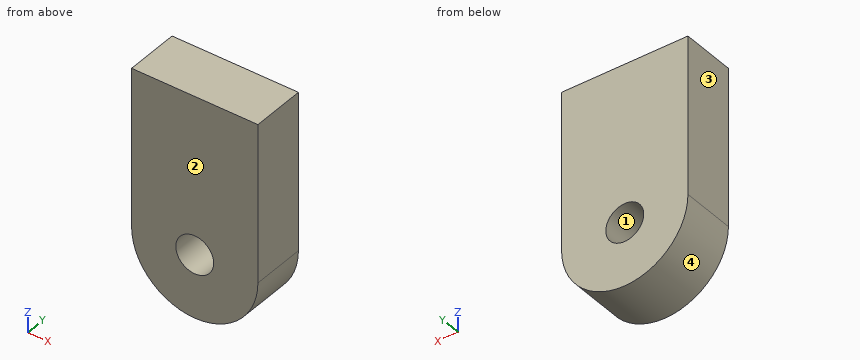
```python
from build123d import *

# Parameters (mm, degrees)
SKETCH1_R           = 2.1
BOSS_EXTRUDE1_DEPTH = 6


with BuildPart() as part:
    # Sketch1 → Boss-Extrude1 (new body)
    with BuildSketch(Plane(origin=(0, 0, 0), x_dir=(1, 0, 0), z_dir=(0, 1, 0))):
        with BuildLine():
            Line((-7, -8.75), (7, -8.75))
            Line((7, -8.75), (7, 8.75))
            ThreePointArc((7, 8.75), (0, 15.75), (-7, 8.75))
            Line((-7, 8.75), (-7, -8.75))
        make_face()
        with Locations((0, 8.75)):
            Circle(SKETCH1_R, mode=Mode.SUBTRACT)
    extrude(amount=BOSS_EXTRUDE1_DEPTH)


solid = part.part
```
For this review, take the finished solid that the model builds, in its own axes (mm). Face numbers are marked on the shaded views. Round coordinates to 2 decimals unless told otherwise and drop trailing zeros. Write each loop counter-clockwise with the first axis right and the second up, starting at its lowest first coordinate (ties: lowest second). Pieces come first, ordered by that corner, then holes. Notation, with made-up numbers: (-11, -14.5) -> (-5, -14.5) arc R31 ccw to (-5, 11.5) -> close; hole circle Ø2 at (-17, -40). An arc over 180 degrees is marked (long way). One line per question, with ' | ' between items. Start each with the question number.
1) Add section D-D (x = -4). Write out the cut boundary in (y, z).
2) Add section A-A (x = 0). Write out the cut boundary in (y, z).
3) Mouldability with a two-part tool opening along X and no side actions: class the marked faces 1, 2, 3 and 4 as +X half, -X half, draft (parallel to the pull), parting line (faces both ways), or undercut.
4) Add section C-C (z = -7.5). Write out the cut boundary in (x, y).
5) Add section B-B (y = 2.65). Write out the cut boundary in (x, z), and give its area (3 significant figures).
6) Wall thickness on line 1 along Z through (x, y) = (0, 4.7); line 2 along X through (y, z) = (4.05, -8.75); line 3 along X through (y, z) = (4.75, -7.75): over which ranges is each line inside the solid? List them lowest first.
7) For pin 1 Ø3 at (x, y) = (3, 4) entering from -Z; pin 2 Ø4 at (x, z) = (0, -8.75) entering from +Y, all flat-tipped, find the tip position at first contact; note any pin that passes through.
Reported:
1) outline: (0, -14.49) -> (6, -14.49) -> (6, 8.75) -> (0, 8.75) -> close
2) outline: (0, -15.75) -> (6, -15.75) -> (6, -10.85) -> (0, -10.85) -> close; (0, -6.65) -> (6, -6.65) -> (6, 8.75) -> (0, 8.75) -> close
3) face 1: undercut | face 2: draft | face 3: -X half | face 4: parting line
4) outline: (-7, 0) -> (-1.69, 0) -> (-1.69, 6) -> (-7, 6) -> close; (1.69, 0) -> (7, 0) -> (7, 6) -> (1.69, 6) -> close
5) outline: (-7, -8.75) arc R7 ccw to (7, -8.75) -> (7, 8.75) -> (-7, 8.75) -> close; hole circle Ø4.2 at (0, -8.75) | area: 308 mm²
6) line 1: z = -15.75 to -10.85, -6.65 to 8.75 | line 2: x = -7 to -2.1, 2.1 to 7 | line 3: x = -7 to -1.85, 1.85 to 7
7) pin 1: stops at z = -15.59 | pin 2: passes through
